from build123d import *

# Parameters (mm, degrees)
SKETCH1_R           = 15
SKETCH1_R_2         = 1.5
SKETCH1_R_3         = 1
BOSS_EXTRUDE1_DEPTH = 1.5
SKETCH2_R           = 5
SKETCH2_R_2         = 3
BOSS_EXTRUDE2_DEPTH = 4


with BuildPart() as part:
    # Sketch1 → Boss-Extrude1 (new body)
    with BuildSketch(Plane.XY):
        with Locations((-39.444879197, 67.794412983)):
            Circle(SKETCH1_R)
        with Locations((-32.949688669, 71.544412983)):
            Circle(SKETCH1_R_2, mode=Mode.SUBTRACT)
        with Locations((-45.940069726, 64.044412983)):
            Circle(SKETCH1_R_2, mode=Mode.SUBTRACT)
        with Locations((-39.444879197, 67.794412983)):
            Circle(SKETCH1_R_3, mode=Mode.SUBTRACT)
        with Locations((-35.694879197, 61.299222454)):
            Circle(SKETCH1_R_2, mode=Mode.SUBTRACT)
        with Locations((-43.194879197, 74.289603511)):
            Circle(SKETCH1_R_2, mode=Mode.SUBTRACT)
    extrude(amount=BOSS_EXTRUDE1_DEPTH)

    # Sketch2 → Boss-Extrude2 (add)
    with BuildSketch(Plane.XY.offset(1.5)):
        with Locations((-39.444879197, 67.794412983)):
            Circle(SKETCH2_R)
        with Locations((-39.444879197, 67.794412983)):
            Circle(SKETCH2_R_2, mode=Mode.SUBTRACT)
    extrude(amount=BOSS_EXTRUDE2_DEPTH)


solid = part.part
Could you check a few things on this model? Use its own coordinates, in mm. A direction names the side the tool comes from. Give positions to 0.01 mm unless a question says otherwise; leave off trailing zeros. Loops run counter-clockwise (first coordinate to the right, second up) from the corner with the lowest first, then second, coordinate; pieces in that order, holes last. Notation, with made-up numbers: M -9,11 L 49,11 A16 ccw 49,20 Z; hole C -17,73 d10. An arc over 180 degrees is marked long. Answer as a JSON object with one key per item and string values.
Q1. Suppose I cut it at C-C, the plane x = -45.5. List the corners of the cut face in (y, z) for me.
Values found:
{"outline": "M 54.07,0 L 62.61,0 L 62.61,1.5 L 54.07,1.5 Z; M 65.48,0 L 81.52,0 L 81.52,1.5 L 65.48,1.5 Z"}
Q2. If I drill on probe 1 along Z at (x, y) = (-52.75, 63); probe 2 along X at (y, z) = (68, 3.4); probe 3 along X at (y, z) = (60.5, 1), over which ranges is the centre line in solid material (lowest first)? Write a range as [from, to].
Values found:
{"probe 1": "z = [0, 1.5]", "probe 2": "x = [-44.44, -42.44], [-36.45, -34.45]", "probe 3": "x = [-52.55, -36.96], [-34.43, -26.34]"}
Q3. If we mould it in two halves opening along Y, with no side actions, what happens to faces 1 (the cylindrical face through (-32.143, 72.809, 0.74)), 2 (the cylindrical face through (-36.757, 72.01, 3.472)), 3 (the flat face through (-36, 68, 5.5))? For each: pulls with the +Y half, pulls with the -Y half, needs draft (parallel to the pull), parting line crosses it, or undercut.
Values found:
{"face 1": "undercut", "face 2": "parting line crosses it", "face 3": "needs draft"}
Q4. Suppose I cut it at B-B, the plane z = 1. List the corners of the cut face in (x, y) for me.
Values found:
{"outline": "C -39.44,67.79 d30; hole C -45.94,64.04 d3; hole C -43.19,74.29 d3; hole C -39.44,67.79 d2; hole C -35.69,61.3 d3; hole C -32.95,71.54 d3"}
Q5. For faces 4 (the cylindrical face through (-32.5, 54.5, 0.7)), 5 (the cylindrical face through (-38.061, 65.133, 3.472)), which set-ups out of +Z, -Z, +X, -X, +Y, -Y let a thin tool reach every point of the face, with its end or its side?
Values found:
{"face 4": "+Z, -Z", "face 5": "+Z"}
Q6. Suppose I cut it at D-D, the plane z = 3.9. List the corners of the cut face in (x, y) for me.
Values found:
{"outline": "C -39.44,67.79 d10; hole C -39.44,67.79 d6"}
Q7. Suppose I cut it at A-A, the plane x = -33.5. List the corners of the cut face in (y, z) for me, plus the area to 3 significant figures.
Values found:
{"outline": "M 54.02,0 L 70.15,0 L 70.15,1.5 L 54.02,1.5 Z; M 72.94,0 L 81.57,0 L 81.57,1.5 L 72.94,1.5 Z", "area": "37.1 mm²"}
Q8. For P1, Ø1, axis at y = 61.5, z = 1.5, coming from the -X side; P2, Ø2, axis at y = 57, z = 2, coming from the +X side; P3, Ø3.5, axis at x = -39.44, y = 67.79, coming from the +Z side, each with a flat end and sliding along its axis, tell me the tip position at first contact or that it passes through.
Values found:
{"P1": "stops at x = -53.28", "P2": "stops at x = -28.2", "P3": "stops at z = 1.5"}
